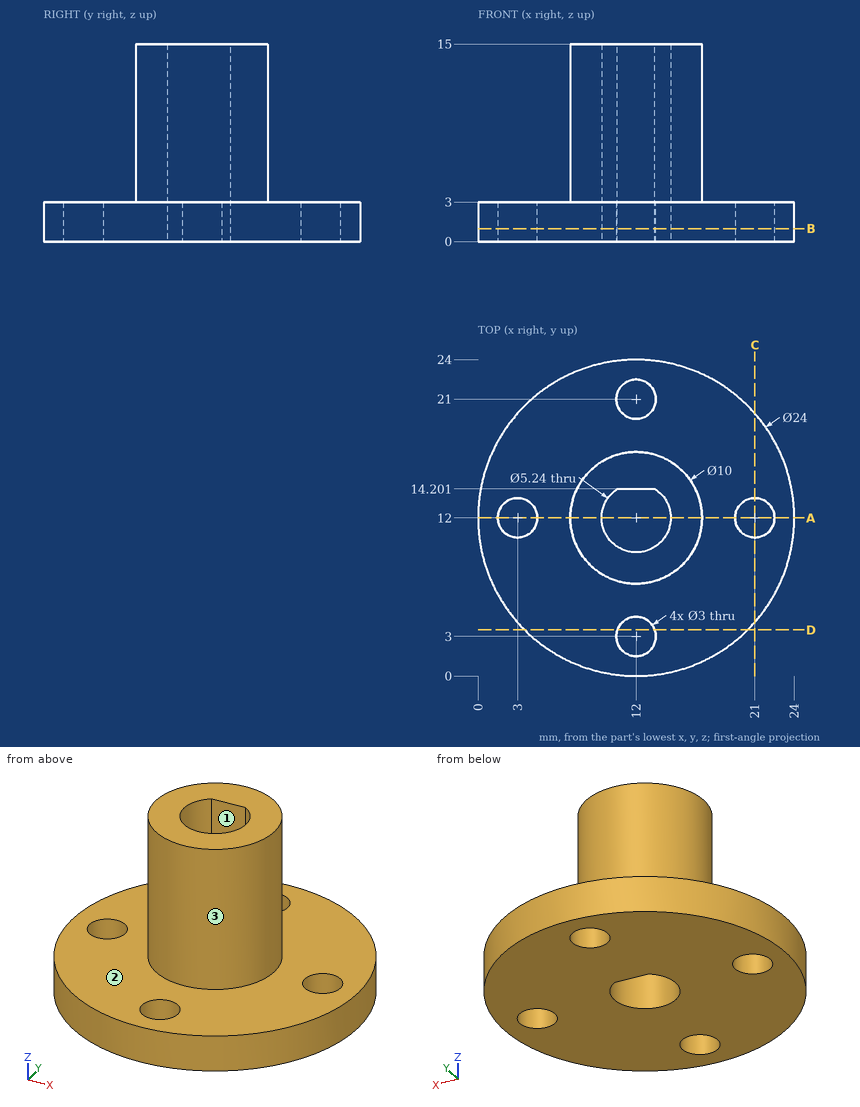
For this review, use the dimensioned drawing (mm, ordinates from the lowest corner) and the shaded views. Round coordinates to 2 decimals unless told otherwise and drop trailing zeros. Write each loop counter-clockwise with the first axis right and the second up, starting at its lowest first coordinate (ties: lowest second). Pieces come first, ordered by that corner, then holes. Notation, with made-up numbers: (22.5, -8.5) -> (28.5, -8.5) arc R26 cw to (28.5, 30.5) -> close; hole circle Ø8 at (76, 77.5). An arc over 180 degrees is marked (long way). Use one line per item in the form item = value.
Q1. Consider section B-B (z = 1). State the section outline as (x, y) points.
Resolved:
outline = circle Ø24 at (12, 12); hole circle Ø3 at (3, 12); hole circle Ø3 at (12, 3); hole circle Ø3 at (12, 21); hole (10.58, 14.2) arc R2.62 ccw (long way) to (13.42, 14.2) -> close; hole circle Ø3 at (21, 12)
Q2. Consider section D-D (y = 3.5). State the section outline as (x, z) points.
Resolved:
outline = (3.53, 0) -> (10.59, 0) -> (10.59, 3) -> (3.53, 3) -> close; (13.41, 0) -> (20.47, 0) -> (20.47, 3) -> (13.41, 3) -> close
Q3. Clearance check with flat-ended pins moving along their axes: pin 1 Ø1.5 at (x, y) = (4, 11) entering from +Z; pin 2 Ø5 at (x, z) = (17, 1.5) entering from -Y; pin 3 Ø0.9 at (x, z) = (11.5, 6) entering from -Y. State where each tip first meets the part, or that it passes through.
Resolved:
pin_1 = 3
pin_2 = 0.26
pin_3 = 7
Q4. Consider section A-A (y = 12). State the section outline as (x, z) points, then the cut area to 3 significant figures.
Resolved:
outline = (0, 0) -> (1.5, 0) -> (1.5, 3) -> (0, 3) -> close; (4.5, 0) -> (9.38, 0) -> (9.38, 15) -> (7, 15) -> (7, 3) -> (4.5, 3) -> close; (14.62, 0) -> (19.5, 0) -> (19.5, 3) -> (17, 3) -> (17, 15) -> (14.62, 15) -> close; (22.5, 0) -> (24, 0) -> (24, 3) -> (22.5, 3) -> close
area = 95.4 mm²
Q5. To check wall thickness, follow probe 1 along Z at (x, y) = (19, 12); probe 2 along X at (y, z) = (13, 7.5); probe 3 along X at (y, z) = (3, 1.5). State the ranges of each line that lie inside material, in increasing order. Write a range as from..to.
Resolved:
probe_1 = 0..3
probe_2 = 7.1..9.58, 14.42..16.9
probe_3 = 4.06..10.5, 13.5..19.94
Q6. Consider section C-C (x = 21). State the section outline as (y, z) points, then the cut area to 3 significant figures.
Resolved:
outline = (4.06, 0) -> (10.5, 0) -> (10.5, 3) -> (4.06, 3) -> close; (13.5, 0) -> (19.94, 0) -> (19.94, 3) -> (13.5, 3) -> close
area = 38.6 mm²
Q7. The part is to be moulded in two halves that separate along Y. For the marked faces 1, 2 and 3, say which applies: released by +Y, released by -Y, zero draft, split by the parting line, or undercut.
Resolved:
face_1 = undercut
face_2 = zero draft
face_3 = split by the parting line
